Autodesk Inventor part; units mm, degrees
ref_plane "YZ Plane" through (0, 0, 0) normal (1, 0, 0) x (0, 1, 0)
ref_plane "XZ Plane" through (0, 0, 0) normal (0, 1, 0) x (-1, 0, 0)
ref_plane "XY Plane" through (0, 0, 0) normal (0, 0, 1) x (1, 0, 0)
sketch "Sketch1" plane through (0, 0, 0) normal (0, 1, 0) x (-1, 0, 0)
  line L0 (0, 0) -> (435, 0)
  line L1 (435, 0) -> (435, -30)
  line L2 (435, -30) -> (0, -30)
  line L3 (0, -30) -> (0, 0)
  dimension "d0" = 435
  dimension "d1" = 30
extrude "Extrusion1" add sketch "Sketch1" along normal blind 5
sketch "Sketch2" plane through (0, 5, 0) normal (0, 1, 0) x (1, 0, 0)
  line L0 (0, 30) -> (-435, 30)
  line L1 (-435, 30) -> (-425, 30)
  line L2 (-425, 30) -> (-420.5, 30)
  line L3 (-420.5, 30) -> (-420.5, 15)
  line L4 (-420.5, 15) -> (-425, 15)
  line L5 (-425, 15) -> (-425, 30)
  line L6 (-420.5, 30) -> (-219.75, 30)
  line L7 (-219.75, 30) -> (-215.25, 30)
  line L8 (-215.25, 30) -> (-215.25, 15)
  line L9 (-215.25, 15) -> (-219.75, 15)
  line L10 (-219.75, 15) -> (-219.75, 30)
  line L11 (-215.25, 30) -> (-14.5, 30)
  line L12 (-14.5, 30) -> (-10, 30)
  line L13 (-10, 30) -> (-10, 15)
  line L14 (-10, 15) -> (-14.5, 15)
  line L15 (-14.5, 15) -> (-14.5, 30)
  point P0 (0, 0)
  dimension "d4" = 10
  dimension "d5" = 4.5
  dimension "d6" = 15
  dimension "d7" = 200.75
  dimension "d8" = 4.5
  dimension "d9" = 15
  dimension "d10" = 200.75
  dimension "d11" = 4.5
  dimension "d12" = 15
extrude "Extrusion2" cut sketch "Sketch2" against normal blind 5
sketch "Sketch3" plane through (0, 5, 0) normal (0, 1, 0) x (1, 0, 0)
  line L0 (-435, 30) -> (-435, 0)
  line L1 (-435, 30) -> (-445, 30)
  line L2 (-445, 30) -> (-445, -290)
  line L3 (-445, -290) -> (-435, -290)
  line L4 (-435, -290) -> (-435, 30)
  line L5 (-435, -290) -> (-420, -290)
  line L6 (-420, -290) -> (-420, 15)
  line L7 (-420, 15) -> (-435, 15)
  line L8 (-435, 15) -> (-435, -290)
  point P0 (0, 0)
  dimension "d15" = 10
  dimension "d16" = 320
  dimension "d17" = 15
  dimension "d18" = 305
extrude "Extrusion3" add sketch "Sketch3" against normal blind 5
fillet "Fillet1" radius 75 1 edges at (-420, 2.5, 0)
sketch "Sketch4" plane through (0, 5, 0) normal (0, 1, 0) x (1, 0, 0)
  line L0 (-10, 15) -> (-14.5, 15)
  line L1 (-14.5, 15) -> (-58.5, 15)
  line L2 (-345, 0) -> (0, 0)
  line L3 (-58.5, 15) -> (-63, 15)
  line L4 (-63, 15) -> (-63, 0)
  line L5 (-63, 0) -> (-58.5, 0)
  line L6 (-58.5, 0) -> (-58.5, 15)
  line L7 (-63, 0) -> (-110.75, 0)
  line L8 (-110.75, 0) -> (-115.25, 0)
  line L9 (-115.25, 0) -> (-115.25, 15)
  line L10 (-115.25, 15) -> (-110.75, 15)
  line L11 (-110.75, 15) -> (-110.75, 0)
  line L12 (-115.25, 0) -> (-163, 0)
  line L13 (-163, 0) -> (-215.25, 0)
  line L14 (-215.25, 0) -> (-219.75, 0)
  line L15 (-163, 0) -> (-167.5, 0)
  line L16 (-167.5, 0) -> (-167.5, 15)
  line L17 (-167.5, 15) -> (-163, 15)
  line L18 (-163, 15) -> (-163, 0)
  line L19 (-217.5, 0) -> (-217.5, 32.2246)
  line L20 (-372, 0) -> (-324.25, 0)
  line L21 (-324.25, 0) -> (-319.75, 0)
  line L22 (-319.75, 0) -> (-319.75, 15)
  line L23 (-319.75, 15) -> (-324.25, 15)
  line L24 (-324.25, 15) -> (-324.25, 0)
  line L25 (-319.75, 0) -> (-272, 0)
  line L26 (-272, 0) -> (-267.5, 0)
  line L27 (-267.5, 0) -> (-267.5, 15)
  line L28 (-267.5, 15) -> (-272, 15)
  line L29 (-272, 15) -> (-272, 0)
  line L30 (-372, 0) -> (-376.5, 0)
  line L31 (-376.5, 0) -> (-376.5, 30)
  line L32 (-376.5, 30) -> (-372, 30)
  line L33 (-372, 30) -> (-372, 0)
  line L34 (-376.5, 30) -> (-372, 30)
  line L35 (-372, 30) -> (-372, 15)
  line L36 (-372, 15) -> (-376.5, 15)
  line L37 (-376.5, 15) -> (-376.5, 30)
  line L38 (-14.5, 15) -> (-459.3643, 15)
  line L39 (-63, 15) -> (-63, 30)
  line L40 (-63, 30) -> (-58.5, 30)
  line L41 (-58.5, 30) -> (-58.5, 15)
  line L42 (-63, 30) -> (-110.75, 30)
  line L43 (-110.75, 30) -> (-115.25, 30)
  line L44 (-115.25, 30) -> (-115.25, 15)
  line L45 (-110.75, 15) -> (-110.75, 30)
  line L46 (-115.25, 30) -> (-163, 30)
  line L47 (-163, 30) -> (-215.25, 30)
  line L48 (-215.25, 30) -> (-219.75, 30)
  line L49 (-163, 30) -> (-167.5, 30)
  line L50 (-167.5, 30) -> (-167.5, 15)
  line L51 (-163, 15) -> (-163, 30)
  line L52 (-267.5, 30) -> (-267.5, 15)
  line L53 (-272, 30) -> (-267.5, 30)
  line L54 (-272, 15) -> (-272, 30)
  line L55 (-319.75, 30) -> (-272, 30)
  line L56 (-319.75, 30) -> (-319.75, 15)
  line L57 (-324.25, 30) -> (-319.75, 30)
  line L58 (-324.25, 15) -> (-324.25, 30)
  line L59 (-372, 30) -> (-324.25, 30)
  line L60 (-372, 30) -> (-376.5, 30)
  line L61 (-324.25, 0) -> (-319.75, 0)
  line L62 (-319.75, 0) -> (-319.75, -4.5)
  line L63 (-319.75, -4.5) -> (-324.25, -4.5)
  line L64 (-324.25, -4.5) -> (-324.25, 0)
  point P0 (-345, 30)
  point P1 (-217.5, 30)
  dimension "d22" = 44
  dimension "d23" = 4.5
  dimension "d24" = 47.75
  dimension "d25" = 4.5
  dimension "d26" = 15
  dimension "d27" = 47.75
  dimension "d28" = 52.25
  dimension "d29" = 4.5
  dimension "d30" = 4.5
  dimension "d31" = 15
  dimension "d38" = 4.5
  dimension "d39" = 30
  dimension "d45" = 4.5
extrude "Extrusion4" cut sketch "Sketch4" against normal blind 5 contours L54 L53 L52 L28 | L50 L47 L51 L17 | L39 L40 L41 L3
sketch "Sketch6" plane through (0, 5, 0) normal (0, 1, 0) x (1, 0, 0)
  line L0 (-420, -75) -> (-420, -290)
  line L1 (-420, -290) -> (-429.75, -290)
  line L2 (-420, -290) -> (-445, -290)
  line L3 (-429.75, -290) -> (-434.25, -290)
  line L4 (-434.25, -290) -> (-434.25, -275)
  line L5 (-434.25, -275) -> (-429.75, -275)
  line L6 (-429.75, -275) -> (-429.75, -290)
  point P0 (0, 0)
  dimension "d40" = 9.75
  dimension "d41" = 4.5
  dimension "d42" = 15
extrude "Extrusion6" cut sketch "Sketch6" against normal blind 5
fillet "Fillet2" radius 1 31 edges at (-10, 2.5, -15) (-14.5, 2.5, -15) (0, 2.5, 0) (0, 2.5, -30) (-14.5, 2.5, -30) (-10, 2.5, -30) (-58.5, 2.5, -30) (-58.5, 2.5, -15) (-63, 2.5, -15) (-63, 2.5, -30) (-163, 2.5, -30) (-167.5, 2.5, -30) (-163, 2.5, -15) (-167.5, 2.5, -15) (-215.25, 2.5, -15) (-219.75, 2.5, -15) (-219.75, 2.5, -30) (-215.25, 2.5, -30) (-272, 2.5, -30) (-267.5, 2.5, -30) (-267.5, 2.5, -15) (-272, 2.5, -15) (-420.5, 2.5, -30) (-425, 2.5, -30) (-420.5, 2.5, -15) (-425, 2.5, -15) (-445, 2.5, -30) (-420, 2.5, 290) (-434.25, 2.5, 275) (-429.75, 2.5, 275) (-445, 2.5, 290)
properties part number "slats_back_over" material "Foam Core Board"
The model under review builds one solid part; all positions refer to its coordinate system, in mm. Round coordinates to 2 decimals unless told otherwise and drop trailing zeros. Loops run counter-clockwise (first coordinate to the right, second up) from the corner with the lowest first, then second, coordinate; pieces in that order, holes last. Notation, with made-up numbers: (29.5, 70.5) -> (78.5, 70.5) arc R28 cw to (78.5, 97.5) -> close; hole circle Ø10 at (59, 36.5). An arc over 180 degrees is marked (long way). One line per question, with ' | ' between items. Start each with the question number.
Item 1: Wall thickness on line 1 along X through (y, z) = (4.05, 253.5); line 2 along Z through (x, y) = (-130, 3.65); line 3 along Z through (x, y) = (-424, 3.8): over which ranges is each line inside the solid? List them lowest first. Write a range as [from, to].
Item 2: Add section B-B, the plane x = -35. Write out the cut boundary in (y, z).
Item 3: Add section A-A, the plane z = 158. Write out the cut boundary in (x, y), then the cut area to 3 significant figures.
Item 4: For pin 1 (1 mm diameter, centred on x = -209, y = 3, fed in from +Z); pin 2 (3 mm diameter, centred on x = -12.5, y = 2.5, fed in from -Z); pin 3 (2 mm diameter, centred on x = -60.5, y = 3, fed in from -Z), all flat-tipped, find the tip position at first contact; note any pin that passes through.
Return value:
1) line 1: x = [-445, -420] | line 2: z = [-30, 0] | line 3: z = [-15, 290]
2) outline: (0, -30) -> (5, -30) -> (5, 0) -> (0, 0) -> close
3) outline: (-445, 0) -> (-420, 0) -> (-420, 5) -> (-445, 5) -> close | area: 125 mm2
4) pin 1: stops at z = 0 | pin 2: stops at z = -15.13 | pin 3: stops at z = -15
